```python
from build123d import *

# Parameters (mm, degrees)
CROQUIS1_R              = 2.5
SALIENTE_EXTRUIR1_DEPTH = 5
SALIENTE_EXTRUIR3_DEPTH = 10
CROQUIS4_W              = 10
CROQUIS4_H              = 20
CORTAR_EXTRUIR1_DEPTH   = 6


with BuildPart() as part:
    # Croquis1 → Saliente-Extruir1 (new body)
    with BuildSketch(Plane(origin=(0, 0, 0), x_dir=(1, 0, 0), z_dir=(0, 1, 0))):
        with BuildLine():
            Line((-71.215351812, -100.39445629), (-71.215351812, -85.39445629))
            Line((-71.215351812, -85.39445629), (128.784648188, -85.39445629))
            Line((128.784648188, -85.39445629), (128.784648188, 64.60554371))
            Line((128.784648188, 64.60554371), (-71.215351812, 64.60554371))
            Line((-71.215351812, 64.60554371), (-71.215351812, 79.60554371))
            Line((-71.215351812, 79.60554371), (-80.302472959, 79.60554371))
            ThreePointArc((-80.302472959, 79.60554371), (-112.63670805, -10.39445629), (-80.302472959, -100.39445629))
            Line((-80.302472959, -100.39445629), (-71.215351812, -100.39445629))
        make_face()
        with Locations((118.784648188, 54.60554371)):
            Circle(CROQUIS1_R, mode=Mode.SUBTRACT)
        with Locations((18.784648188, -75.39445629)):
            Circle(CROQUIS1_R, mode=Mode.SUBTRACT)
        with Locations((118.784648188, -75.39445629)):
            Circle(CROQUIS1_R, mode=Mode.SUBTRACT)
        with Locations((18.784648188, 54.60554371)):
            Circle(CROQUIS1_R, mode=Mode.SUBTRACT)
    extrude(amount=SALIENTE_EXTRUIR1_DEPTH)

    # Croquis3 → Saliente-Extruir3 (add)
    with BuildSketch(Plane(origin=(0, 5, 0), x_dir=(1, 0, 0), z_dir=(0, 1, 0))):
        with BuildLine():
            Line((-101.63670805, -10.39445629), (-97.63670805, -10.39445629))
            ThreePointArc((-97.63670805, -10.39445629), (-89.972723776, 2.089729896), (-75.371721661, 0.90554371))
            Line((-75.371721661, 0.90554371), (-69.625640995, 0.90554371))
            ThreePointArc((-69.625640995, 0.90554371), (-89.62840201, 6.579040801), (-101.63670805, -10.39445629))
        make_face()
        with BuildLine():
            ThreePointArc((-75.371721661, -21.69445629), (-89.972723776, -22.878642476), (-97.63670805, -10.39445629))
            Line((-97.63670805, -10.39445629), (-101.63670805, -10.39445629))
            ThreePointArc((-101.63670805, -10.39445629), (-89.62840201, -27.367953381), (-69.625640995, -21.69445629))
            Line((-69.625640995, -21.69445629), (-75.371721661, -21.69445629))
        make_face()
        with BuildLine():
            ThreePointArc((-71.69057897, -17.69445629), (-73.335140348, -19.874841455), (-75.371721661, -21.69445629))
            Line((-75.371721661, -21.69445629), (-69.625640995, -21.69445629))
            ThreePointArc((-69.625640995, -21.69445629), (-68.273800946, -19.7742796), (-67.183440897, -17.69445629))
            Line((-67.183440897, -17.69445629), (-71.69057897, -17.69445629))
        make_face()
        with BuildLine():
            Line((-62.63670805, 0.90554371), (-69.625640995, 0.90554371))
            ThreePointArc((-69.625640995, 0.90554371), (-68.273800946, -1.01463298), (-67.183440897, -3.09445629))
            Line((-67.183440897, -3.09445629), (-66.63670805, -3.09445629))
            Line((-66.63670805, -3.09445629), (-66.63670805, -4.478376507))
            ThreePointArc((-66.63670805, -4.478376507), (-65.8884687, -7.39445629), (-65.63670805, -10.39445629))
            ThreePointArc((-65.63670805, -10.39445629), (-65.8884687, -13.39445629), (-66.63670805, -16.310536073))
            Line((-66.63670805, -16.310536073), (-66.63670805, -17.69445629))
            Line((-66.63670805, -17.69445629), (-67.183440897, -17.69445629))
            ThreePointArc((-67.183440897, -17.69445629), (-68.273800946, -19.7742796), (-69.625640995, -21.69445629))
            Line((-69.625640995, -21.69445629), (-62.63670805, -21.69445629))
            Line((-62.63670805, -21.69445629), (-62.63670805, 0.90554371))
        make_face()
        with BuildLine():
            Line((-66.63670805, -4.478376507), (-66.63670805, -10.39445629))
            Line((-66.63670805, -10.39445629), (-66.63670805, -16.310536073))
            ThreePointArc((-66.63670805, -16.310536073), (-65.8884687, -13.39445629), (-65.63670805, -10.39445629))
            ThreePointArc((-65.63670805, -10.39445629), (-65.8884687, -7.39445629), (-66.63670805, -4.478376507))
        make_face()
        with BuildLine():
            Line((-69.625640995, 0.90554371), (-75.371721661, 0.90554371))
            ThreePointArc((-75.371721661, 0.90554371), (-73.335140348, -0.914071125), (-71.69057897, -3.09445629))
            Line((-71.69057897, -3.09445629), (-67.183440897, -3.09445629))
            ThreePointArc((-67.183440897, -3.09445629), (-68.273800946, -1.01463298), (-69.625640995, 0.90554371))
        make_face()
    extrude(amount=SALIENTE_EXTRUIR3_DEPTH)

    # Croquis4 → Cortar-Extruir1 (cut)
    with BuildSketch(Plane(origin=(0, 5, 0), x_dir=(1, 0, 0), z_dir=(0, 1, 0))):
        with Locations((-32.63670805, -10.39445629)):
            Rectangle(CROQUIS4_W, CROQUIS4_H)
    extrude(amount=-CORTAR_EXTRUIR1_DEPTH, mode=Mode.SUBTRACT)


solid = part.part
```
Model file for the job. Use its own axes, mm. A direction names the side the tool comes from. Give positions to 0.01 mm unless a question says otherwise; leave off trailing zeros. Write each loop counter-clockwise with the first axis right and the second up, starting at its lowest first coordinate (ties: lowest second). Pieces come first, ordered by that corner, then holes. Notation, with made-up numbers: (-39, -16.5) -> (-8, -16.5) arc R5 ccw to (-8, -10.5) -> close; hole circle Ø1 at (51, -37). An arc over 180 degrees is marked (long way). Use CSV: the item, a comma, the result in double quotes. Start each with the question number.
1) Drill centre lines: L1, parallel to Z at x = -60.5, y = 2.5; L2, parallel to Y at x = 117, z = -64.5; L3, parallel to X at y = 12.5, z = 18.5. Where is each one in solid material? Low to high.
2) Two-plate mould, pull along X, no slides. Class faces 1 (the flat face through (-71.215, 2, -72)), 2 (the flat face through (-66, 10, -0.906)), 3 (the flat face through (-82, 5, 10)): released by +X, released by -X, zero draft, split by the parting line, or undercut.
3) Tool access for faces 4 (the flat face through (-66.637, 10, 10)), 5 (the flat face through (-33, 3, 20.394)), 6 (the flat face through (30, 2, -64.606)), 7 (the flat face through (27, 2, 85.394)): list every direction of +Z, -Z, +X, -X, +Y, -Y with a clear straight run to the whole face (end or side of a thin tool).
4) Pin check, flat tips, straight feed: P1, Ø6, axis at x = 18.78, z = -54.61, coming from the -Y side; P2, Ø10, axis at x = 67.5, z = -30.5, coming from the +Y side; P3, Ø5.5, axis at x = -10, y = 2.5, coming from the -Z side; P4, Ø4, axis at y = 1.5, z = 95, coming from the +X side. Stop position of each tip, or through.
5) Cut at A-A on y = 8.5. List the corners of the cut face in (x, z).
6) Cut at D-D on z = -30. List the corners of the cut face in (x, y) (3 decimals), plus the area to 3 significant figures.
7) Cut at B-B on z = 13.5. List the corners of the cut face in (x, y), plus the area to 3 significant figures.
8) Cut at C-C on x = 84. List the corners of the cut face in (y, z).
Final values:
1,L1,"z = -64.61 to 85.39"
1,L2,"y = 0 to 5"
1,L3,"x = -99.71 to -95.05, -72.22 to -62.64"
2,face 1,"released by +X"
2,face 2,"zero draft"
2,face 3,"undercut"
3,face 4,"+Y"
3,face 5,"+Y, -Y"
3,face 6,"-Z, +X, +Y, -Y"
3,face 7,"+Z, +X, +Y, -Y"
4,P1,"stops at y = 0"
4,P2,"stops at y = 5"
4,P3,"stops at z = -64.61"
4,P4,"stops at x = -71.22"
5,outline,"(-69.63, -0.91) -> (-62.64, -0.91) -> (-62.64, 21.69) -> (-69.63, 21.69) arc R18 ccw (long way) to start; hole (-71.69, 3.09) -> (-66.64, 3.09) -> (-66.64, 17.69) -> (-71.69, 17.69) arc R14 ccw (long way) to start"
6,outline,"(-106.745, 0) -> (128.785, 0) -> (128.785, 5) -> (-106.745, 5) -> close"
6,area,"1,180 mm2"
7,outline,"(-112.6, 0) -> (-37.64, 0) -> (-37.64, 5) -> (-62.64, 5) -> (-62.64, 15) -> (-66.64, 15) -> (-66.64, 5) -> (-97.29, 5) -> (-97.29, 15) -> (-101.37, 15) -> (-101.37, 5) -> (-112.6, 5) -> close; (-27.64, 0) -> (128.78, 0) -> (128.78, 5) -> (-27.64, 5) -> close"
7,area,"1,240 mm2"
8,outline,"(0, -64.61) -> (5, -64.61) -> (5, 85.39) -> (0, 85.39) -> close"
